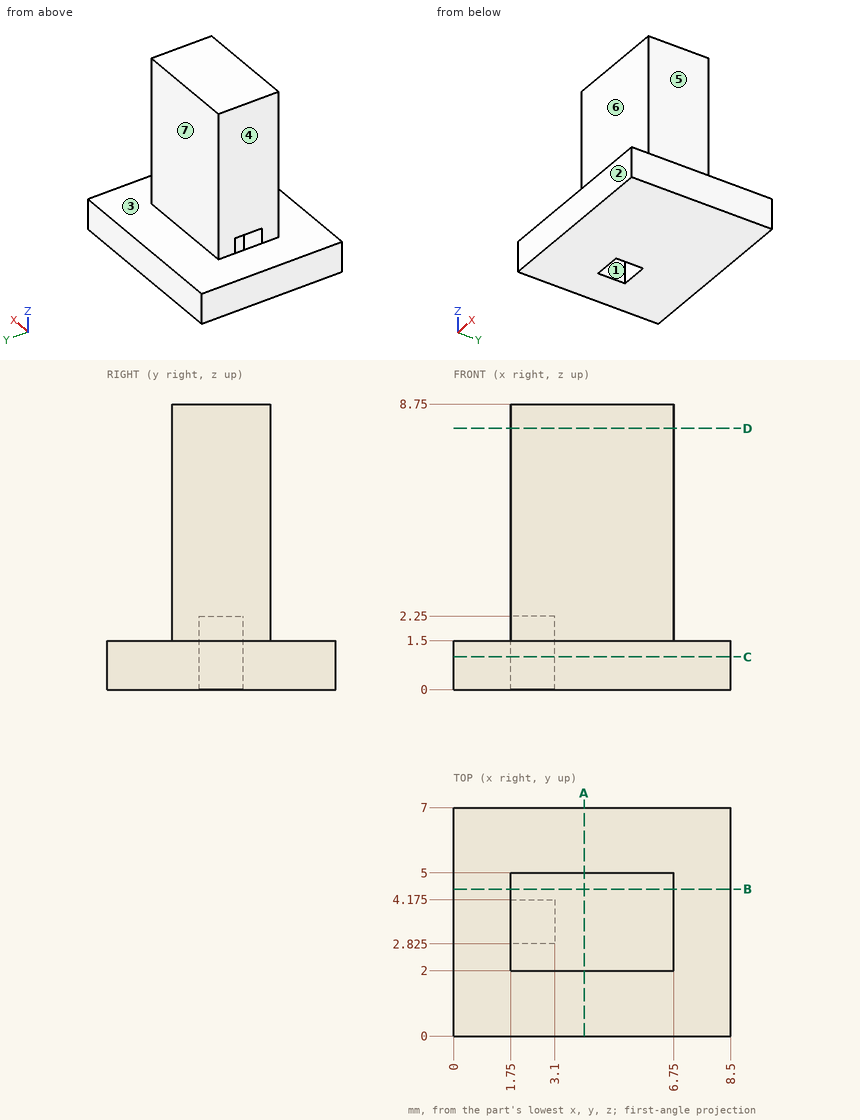
Print and shaded views of the part. All mm, measured from the part's lowest x, y and z. A direction names the side the tool comes from. Coordinates: 2 decimals unless noted, no trailing zeros. Loops run counter-clockwise (first coordinate to the right, second up) from the corner with the lowest first, then second, coordinate; pieces in that order, holes last. Notation, with made-up numbers: (76.5, -30.5) - (130.5, -30.5) arc R29 ccw to (130.5, -5.5) - close; hole circle Ø11 at (59.25, -13.75). An arc over 180 degrees is marked (long way). Write item = value, one per line. Start each with the question number.
Item 1: Flat gauge pins, fed straight in: pin 1 Ø2.5 at (y, z) = (3.5, 6.5) entering from -X; pin 2 Ø1.5 at (y, z) = (3.5, 4.5) entering from +X; pin 3 Ø4 at (x, z) = (2.5, 4) entering from -Y. Where does each tip first touch, or does it go through?
Item 2: Wall check: L1, parallel to X at y = 4.5, z = 7.75; L2, parallel to Y at x = 6.25, z = 4.5; L3, parallel to X at y = 3, z = 0.75. Give the ranges that are in metal, low to high. Write a range as from..to.
Item 3: Cut at D-D, the plane z = 8. Give the cut face in (x, y), and give its area (3 significant figures).
Item 4: Cut at B-B, the plane y = 4.5. Give the cut face in (x, z).
Item 5: 3-axis set-ups, long thin cutter, end or side, ignore diameter. For the marked faces 4, 5, 6 and 7: which of +Z, -Z, +X, -X, +Y, -Y reach the whole face in a straight line?
Item 6: Cut at A-A, the plane x = 4. Give the cut face in (y, z), and give its area (4 significant figures).
Item 7: Mould opens along Y. For the marked faces 1, 2 and 3 say: released by +Y, released by -Y, zero draft, split by the parting line, or undercut.
Item 8: Cut at C-C, the plane z = 1. Give the cut face in (x, y) (3 decimals), and give its area (3 significant figures).
The answers:
q1.pin_1 = 1.75
q1.pin_2 = 6.75
q1.pin_3 = 2
q2.L1 = 1.75..6.75
q2.L2 = 2..5
q2.L3 = 0..1.75, 3.1..8.5
q3.outline = (1.75, 2) - (6.75, 2) - (6.75, 5) - (1.75, 5) - close
q3.area = 15.0 mm2
q4.outline = (0, 0) - (8.5, 0) - (8.5, 1.5) - (6.75, 1.5) - (6.75, 8.75) - (1.75, 8.75) - (1.75, 1.5) - (0, 1.5) - close
q5.face_4 = +Z, -X, +Y, -Y
q5.face_5 = +Z, +X, +Y, -Y
q5.face_6 = +Z, +X, -X, -Y
q5.face_7 = +Z, +X, -X, +Y
q6.outline = (0, 0) - (7, 0) - (7, 1.5) - (5, 1.5) - (5, 8.75) - (2, 8.75) - (2, 1.5) - (0, 1.5) - close
q6.area = 32.25 mm2
q7.face_1 = undercut
q7.face_2 = released by -Y
q7.face_3 = zero draft
q8.outline = (0, 0) - (8.5, 0) - (8.5, 7) - (0, 7) - close; hole (1.75, 2.825) - (3.1, 2.825) - (3.1, 4.175) - (1.75, 4.175) - close
q8.area = 57.7 mm2
